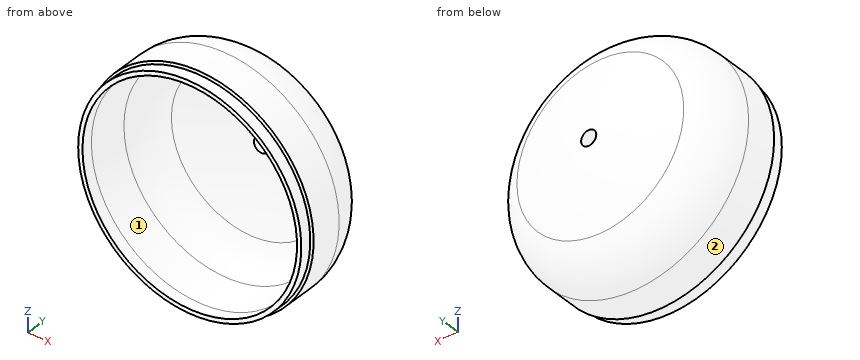
```python
from build123d import *


with BuildPart() as part:
    # Sketch1 → Revolve2 (revolve)
    with BuildSketch(Plane.XY):
        with BuildLine():
            Line((-63.5, 7.0880256), (-63.5, 25.209576395))
            ThreePointArc((-63.5, 25.209576395), (-58.831621889, 40.085351805), (-46.500676471, 49.626328344))
            ThreePointArc((-46.500676471, 49.626328344), (-25.692788323, 55.467905735), (-4.2164, 57.8880256))
            Line((-4.2164, 57.8880256), (-4.2164, 50.899373851))
            ThreePointArc((-4.2164, 50.899373851), (-24.461267699, 48.591399426), (-44.076470588, 43.075492455))
            ThreePointArc((-44.076470588, 43.075492455), (-53.099113577, 36.09429011), (-56.515, 25.209576395))
            Line((-56.515, 25.209576395), (-59.840452163, 6.35))
            Line((-59.840452163, 6.35), (-59.840452163, 0))
            Line((-59.840452163, 0), (-62.221702163, 0))
            Line((-62.221702163, 0), (-62.221702163, 6.35))
            Line((-62.221702163, 6.35), (-63.5, 7.0880256))
        make_face()
    revolve(axis=Axis((0, 127.060987048, 0), (0, -1, 0)))


solid = part.part
```
Design review of the part built by this model. Coordinates are the model's own, in mm. Face numbers are marked on the shaded views. Coordinates: 2 decimals unless noted, no trailing zeros. Write each loop counter-clockwise with the first axis right and the second up, starting at its lowest first coordinate (ties: lowest second). Pieces come first, ordered by that corner, then holes.
1) Insertion check: pin 1 (3 mm diameter, centred on x = -18, z = 39, fed in from -Y); pin 2 (2 mm diameter, centred on x = -46.5, y = 39.5, fed in from +Z); pin 3 (13.5 mm diameter, centred on x = 0, z = 0, fed in from -Y). Each pin has a flat end and moves straight along its axis. Give the tip position at first contact, or say it passes through.
2) Add section D-D (y = 28). Write out the cut boundary in (x, z), plus the area to 3 significant figures.
3) Mouldability with a two-part tool opening along X and no side actions: class the marked faces 1 and 2 as +X half, -X half, draft (parallel to the pull), parting line (faces both ways), or undercut.
4) To check wall thickness, follow L1, parallel to Z at x = 0, y = 1.75; L2, parallel to X at y = 7, z = 33; L3, parallel to X at y = 36, z = 38.5. State the ranges of each line that lie inside material, in increasing order.
5) Add section C-C (y = 11). Write out the cut boundary in (x, z).
Check result:
1. pin 1: stops at y = 42.93
1. pin 2: stops at z = 38.27
1. pin 3: stops at y = 50.79
2. outline: circle Ø126.7 at (0, 0); hole circle Ø112.62 at (0, 0)
2. area: 2,650 mm2
3. face 1: undercut
3. face 2: parting line
4. L1: z = -62.22 to -59.84, 59.84 to 62.22
4. L2: x = -54.07 to -49.78, 49.78 to 54.07
4. L3: x = -47.52 to -36.66, 36.66 to 47.52
5. outline: circle Ø127 at (0, 0); hole circle Ø118.04 at (0, 0)
